Source: three-view drawing plus pictorial views. Frame: mm from the lowest corner of the part. A direction names the side the tool comes from. Round coordinates to 2 decimals unless told otherwise and drop trailing zeros. Write each loop counter-clockwise with the first axis right and the second up, starting at its lowest first coordinate (ties: lowest second). Pieces come first, ordered by that corner, then holes. Notation, with made-up numbers: M 55,-39.5 L 94,-39.5 A7 ccw 94,-27.5 Z; hole C 82.25,15.25 d1. An arc over 180 degrees is marked long. Answer in a Markdown table with one row per item.
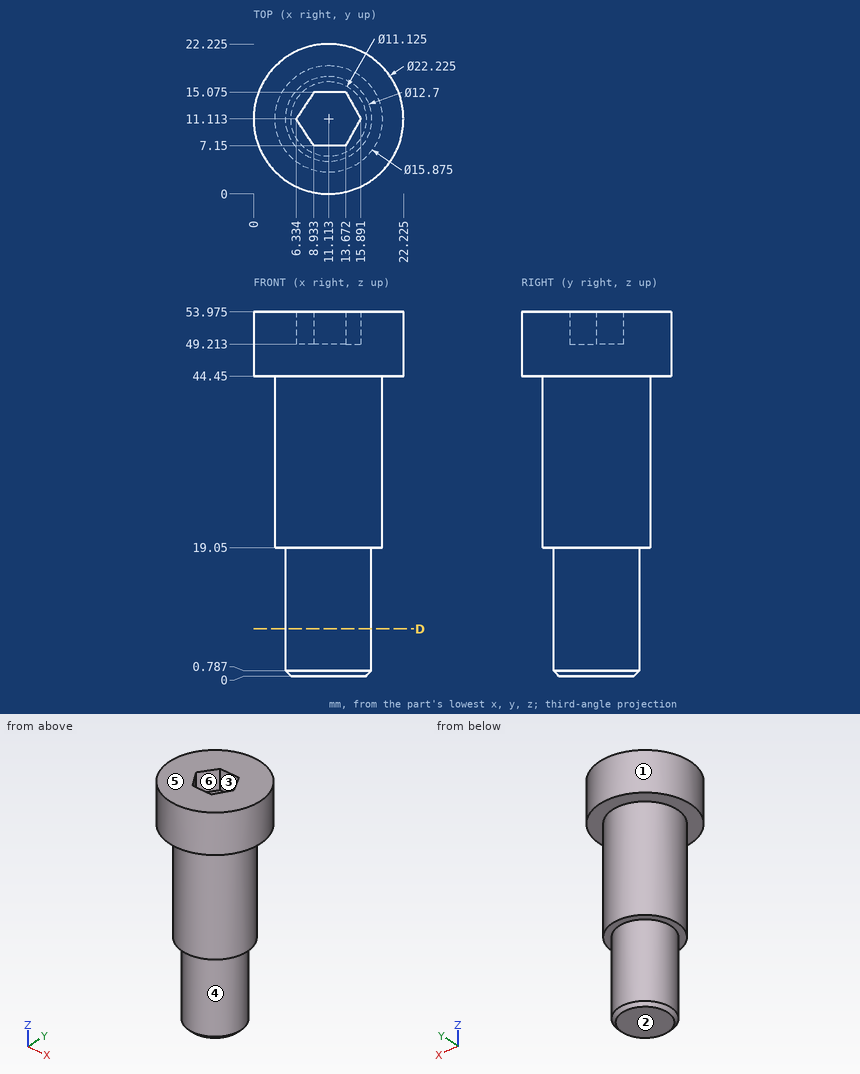
Q1. Contact query for flat-ended pins moving along their axis: pin 1 Ø12 at (y, z) = (14, 17.5) entering from +X; pin 2 Ø8 at (x, y) = (19, 12) entering from -Z; pin 3 Ø2 at (x, z) = (2.5, 47.5) entering from -Y; pin 4 Ø3 at (x, y) = (5, 2.5) entering from -Z. Output: stop coordinate, or through.
Solutions:
| item | result |
|---|---|
| pin 1 | stops at x = 19.05 |
| pin 2 | stops at z = 0 |
| pin 3 | stops at y = 3.02 |
| pin 4 | stops at z = 44.45 |
Q2. Pull-direction query (X, two-part tool) for the marked faces 1, 2 and 3; classes: pulls with the +X half, pulls with the -X half, needs draft (parallel to the pull), parting line crosses it, or undercut.
Solutions:
| item | result |
|---|---|
| face 1 | parting line crosses it |
| face 2 | needs draft |
| face 3 | undercut |
Q3. Material intervals for probe 1 along X at (y, z) = (11.5, 26.5) (1 decimal); probe 2 along X at (y, z) = (8.75, 49.5) (1 decimal); probe 3 along Z at (x, y) = (9, 10.5), sorted ascending.
Solutions:
| item | result |
|---|---|
| probe 1 | x = 3.2 to 19 |
| probe 2 | x = 0.3 to 7.9, 14.6 to 22 |
| probe 3 | z = 0 to 49.21 |
Q4. Access query for the marked faces 4, 5 and 6. Directions: +Z, -Z, +X, -X, +Y, -Y. A direction counts if a zero-diameter tool reaches every point of the face in a straight line with its end or side. Return the directions, or none.
Solutions:
| item | result |
|---|---|
| face 4 | -Z |
| face 5 | +Z, +X, -X, +Y, -Y |
| face 6 | +Z |
Q5. Section D-D (z = 7). Return loops of the section in (x, y).
Solutions:
| item | result |
|---|---|
| outline | C 11.11,11.11 d12.7 |
